Verification items for the finished model (mm, model axes). Give positions to 0.01 mm unless a question says otherwise; leave off trailing zeros. Order: outer loops, then holes, each group sorted by start corner. A loop starts at its lowest first (then second) coordinate and runs counter-clockwise, first axis right, second up. Notation, with made-up numbers: (59, 4.25) -> (108, 4.25) arc R16 ccw to (108, 18.25) -> close; hole circle Ø7 at (87.5, -26). An arc over 180 degrees is marked (long way). Return JSON: item names as keys, results as strings. Group by question number.
(1) Cross-section at C-C on x = 295. Enter the section's corners in (y, z), then the cut area to 3 significant figures.
(2) Depth check by flat-ended pin: pin 1 Ø3 at (x, z) = (170.18, -170.18) entering from -Y; pin 2 Ø4.5 at (x, z) = (335.28, -252.73) entering from +Y; pin 3 Ø0.5 at (y, z) = (-1, -95.5) entering from +X; pin 4 Ø0.8 at (x, y) = (266.5, -0.5) entering from +Z. Enter the tip coordinate at first touch or a pass-through.
(3) Thickness scan on line 1 along X through (y, z) = (-1.1, -5.08); line 2 along X through (y, z) = (-0.85, -170.18); line 3 along X through (y, z) = (-0.8, -252.73). Record the ranges inside material, lowest first.
(4) Cross-section at B-B on z = -294.5. Enter the section's corners in (x, y).
(5) Cross-section at A-A on y = -1.05. State how many separate pieces and enclosed holes the cut face has, then the cut area to 3 significant figures.
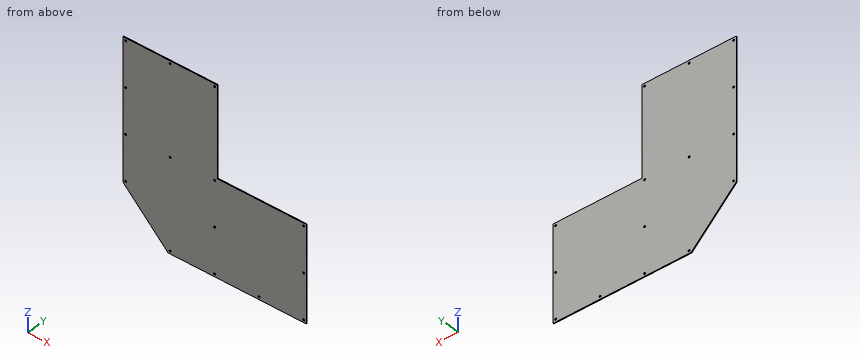
from build123d import *

# Parameters (mm, degrees)
BASE_FLANGE1_DEPTH              = 1.5875
F_29_0_136_DIAMETER_HOLE1_D     = 3.4544
F_29_0_136_DIAMETER_HOLE1_DEPTH = 6.35
F_29_0_136_DIAMETER_HOLE1_TIP   = 1.037806461


# Sheet-metal steps are written as plain solids
with BuildPart() as part:
    # Sketch1 → Base-Flange1 (new body)
    with BuildSketch(Plane(origin=(0, 0, 0), x_dir=(1, 0, 0), z_dir=(0, 1, 0))):
        Polygon((0, 0), (0, 256.54), (83.82, 340.36), (340.36, 340.36), (340.36, 165.1), (175.26, 165.1), (175.26, 0), align=None)
    extrude(amount=-BASE_FLANGE1_DEPTH)

    # #29 (0.136) Diameter Hole1
    with Locations(Plane(origin=(0, 0, 0), x_dir=(1, 0, 0), z_dir=(0, 1, 0))):
        with Locations((5.08, 5.08), (335.28, 170.18), (87.63, 5.08), (170.18, 5.08), (5.08, 87.63), (5.08, 170.18), (5.08, 252.73), (335.28, 252.73), (335.28, 335.28), (252.73, 335.28), (170.18, 335.28), (87.63, 335.28), (170.18, 170.18), (87.63, 170.18), (170.18, 252.73)):
            Hole(F_29_0_136_DIAMETER_HOLE1_D / 2, depth=F_29_0_136_DIAMETER_HOLE1_DEPTH)
            with Locations((0, 0, -(F_29_0_136_DIAMETER_HOLE1_DEPTH + F_29_0_136_DIAMETER_HOLE1_TIP / 2))):  # 118° drill point
                Cone(0, F_29_0_136_DIAMETER_HOLE1_D / 2, F_29_0_136_DIAMETER_HOLE1_TIP, mode=Mode.SUBTRACT)


solid = part.part
Verdict:
{
 "1": {"outline": "(-1.59, -340.36) -> (0, -340.36) -> (0, -165.1) -> (-1.59, -165.1) -> close", "area": "278 mm²"},
 "2": {"pin 1": "through", "pin 2": "y = 0", "pin 3": "x = 175.26", "pin 4": "z = -165.1"},
 "3": {"line 1": "0 to 3.35, 6.81 to 85.9, 89.36 to 168.45, 171.91 to 175.26", "line 2": "0 to 3.35, 6.81 to 85.9, 89.36 to 168.45, 171.91 to 333.55, 337.01 to 340.36", "line 3": "0 to 3.35, 6.81 to 168.45, 171.91 to 333.55, 337.01 to 340.36"},
 "4": {"outline": "(37.96, -1.59) -> (340.36, -1.59) -> (340.36, 0) -> (37.96, 0) -> close"},
 "5": {"separate pieces": "1", "enclosed holes": "15", "area": "84,900 mm²"}
}
